from build123d import *

# Parameters (mm, degrees)
SKETCH1_R           = 14
BOSS_EXTRUDE1_DEPTH = 22
SKETCH2_R           = 12
CUT_EXTRUDE1_DEPTH  = 15
SKETCH3_R           = 17.036826926
SKETCH3_R_2         = 13
CUT_EXTRUDE2_DEPTH  = 15
SKETCH4_R           = 15.163293939
CUT_EXTRUDE3_DEPTH  = 10
SKETCH5_R           = 16.994892588
SKETCH5_R_2         = 4.5
CUT_EXTRUDE4_DEPTH  = 2
SKETCH8_R           = 3.6
CUT_EXTRUDE5_DEPTH  = 7
CIRPATTERN1_COUNT   = 4
SKETCH11_R          = 5.620004384
CUT_EXTRUDE6_DEPTH  = 0.75
SKETCH12_R          = 1.5
CUT_EXTRUDE7_DEPTH  = 18
SKETCH13_R          = 8.375
SKETCH13_R_2        = 4.775
CUT_EXTRUDE8_DEPTH  = 3
FILLET1_SIZE        = 2.75
FILLET2_SIZE        = 3
SKETCH14_W          = 4
SKETCH14_H          = 4.217169846
CUT_EXTRUDE10_DEPTH = 5
CIRPATTERN3_COUNT   = 14
CIRPATTERN3_ANGLE   = 334.282
SKETCH16_R          = 0.75
CUT_EXTRUDE11_DEPTH = 6


with BuildPart() as part:
    # Sketch1 → Boss-Extrude1 (new body)
    with BuildSketch(Plane.XY):
        Circle(SKETCH1_R)
    extrude(amount=BOSS_EXTRUDE1_DEPTH)

    # Sketch2 → Cut-Extrude1 (cut)
    with BuildSketch(Plane(origin=(0, 0, 0), x_dir=(-1, 0, 0), z_dir=(0, 0, -1))):
        Circle(SKETCH2_R)
    extrude(amount=-CUT_EXTRUDE1_DEPTH, mode=Mode.SUBTRACT)

    # Sketch3 → Cut-Extrude2 (cut)
    with BuildSketch(Plane(origin=(0, 0, 0), x_dir=(-1, 0, 0), z_dir=(0, 0, -1))):
        Circle(SKETCH3_R)
        Circle(SKETCH3_R_2, mode=Mode.SUBTRACT)
    extrude(amount=-CUT_EXTRUDE2_DEPTH, mode=Mode.SUBTRACT)

    # Sketch4 → Cut-Extrude3 (cut)
    with BuildSketch(Plane(origin=(0, 0, 0), x_dir=(-1, 0, 0), z_dir=(0, 0, -1))):
        Circle(SKETCH4_R)
    extrude(amount=-CUT_EXTRUDE3_DEPTH, mode=Mode.SUBTRACT)

    # Sketch5 → Cut-Extrude4 (cut)
    with BuildSketch(Plane.XY.offset(22)):
        Circle(SKETCH5_R)
        Circle(SKETCH5_R_2, mode=Mode.SUBTRACT)
    extrude(amount=-CUT_EXTRUDE4_DEPTH, mode=Mode.SUBTRACT)

    # Sketch8 → Cut-Extrude5 (cut)
    with BuildSketch(Plane.XY.offset(20)):
        with Locations((0, 8.375)):
            Circle(SKETCH8_R)
    cut_extrude5 = extrude(amount=-CUT_EXTRUDE5_DEPTH, mode=Mode.SUBTRACT)

    # CirPattern1: Cut-Extrude5 ×4 about axis
    cirpattern1_axis = Axis((0, 0, 0), (0, 0, 1))
    for i in range(1, CIRPATTERN1_COUNT):
        add(cut_extrude5.rotate(cirpattern1_axis, i * 360 / CIRPATTERN1_COUNT), mode=Mode.SUBTRACT)

    # Sketch7 → Cut-Revolve2 (revolve, cut)
    with BuildSketch(Plane(origin=(0, 0, 0), x_dir=(1, 0, 0), z_dir=(0, 1, 0))):
        with BuildLine():
            Line((-14, -16), (-16.211067118, -22.850526422))
            Line((-16.211067118, -22.850526422), (-8.5, -20))
            add(Edge.make_bspline(
                [(-8.5, -20), (-12.342847144, -17.893785877), (-14, -16)],
                knots=[0, 0, 0, 1, 1, 1], degree=2))
        make_face()
    revolve(axis=Axis((0, 0, 9.142490177), (0, 0, 1)), mode=Mode.SUBTRACT)

    # Sketch11 → Cut-Extrude6 (cut)
    with BuildSketch(Plane.XY.offset(22)):
        Circle(SKETCH11_R)
    extrude(amount=-CUT_EXTRUDE6_DEPTH, mode=Mode.SUBTRACT)

    # Sketch12 → Cut-Extrude7 (cut)
    with BuildSketch(Plane.XY.offset(21.25)):
        Circle(SKETCH12_R)
    extrude(amount=-CUT_EXTRUDE7_DEPTH, mode=Mode.SUBTRACT)

    # Sketch13 → Cut-Extrude8 (cut)
    with BuildSketch(Plane(origin=(0, 0, 15), x_dir=(-1, 0, 0), z_dir=(0, 0, -1))):
        Circle(SKETCH13_R)
        Circle(SKETCH13_R_2, mode=Mode.SUBTRACT)
    extrude(amount=-CUT_EXTRUDE8_DEPTH, mode=Mode.SUBTRACT)

    # Fillet1
    fillet1_edges = [part.edges().sort_by_distance(p)[0] for p in [
        (4.775, 0, 15),
    ]]
    chamfer(fillet1_edges, length=FILLET1_SIZE)

    # Fillet2
    # the kernel refuses this chamfer: 3 mm, written as the material it takes off along each edge
    with BuildSketch(Plane(origin=(0, 0, 15), x_dir=(-0.4688986407455129, 0.8832519825661364, 0), z_dir=(-0.8832519825661364, -0.4688986407455129, 0))) as fillet2_piece_1_section:
        Polygon((8.375, -FILLET2_SIZE), (8.375 + FILLET2_SIZE, 0), (8.375, 0), align=None)
    fillet2_piece_1 = revolve(axis=Axis((0, 0, 15), (0, 0, -1)), revolution_arc=145.925657294, mode=Mode.PRIVATE)
    fillet2_piece_1 = split(fillet2_piece_1, bisect_by=Plane(origin=(6.988160105, 6.988160105, 18), z_dir=(0, 0, -1)), keep=Keep.TOP, mode=Mode.PRIVATE)
    add(fillet2_piece_1, mode=Mode.SUBTRACT)
    with BuildSketch(Plane(origin=(0, 0, 15), x_dir=(0.4688986407455169, -0.8832519825661342, 0), z_dir=(0.8832519825661342, 0.4688986407455169, 0))) as fillet2_piece_2_section:
        Polygon((8.375, -FILLET2_SIZE), (8.375 + FILLET2_SIZE, 0), (8.375, 0), align=None)
    fillet2_piece_2 = revolve(axis=Axis((0, 0, 15), (0, 0, -1)), revolution_arc=145.925657294, mode=Mode.PRIVATE)
    fillet2_piece_2 = split(fillet2_piece_2, bisect_by=Plane(origin=(-6.988160104, -6.988160104, 18), z_dir=(0, 0, -1)), keep=Keep.TOP, mode=Mode.PRIVATE)
    add(fillet2_piece_2, mode=Mode.SUBTRACT)
    with BuildSketch(Plane(origin=(0, 0, 15), x_dir=(0.8832519825661352, 0.4688986407455149, 0), z_dir=(-0.4688986407455149, 0.8832519825661352, 0))) as fillet2_piece_3_section:
        Polygon((8.375, -FILLET2_SIZE), (8.375 + FILLET2_SIZE, 0), (8.375, 0), align=None)
    fillet2_piece_3 = revolve(axis=Axis((0, 0, 15), (0, 0, -1)), revolution_arc=145.925657294, mode=Mode.PRIVATE)
    fillet2_piece_3 = split(fillet2_piece_3, bisect_by=Plane(origin=(6.988160105, -6.988160105, 18), z_dir=(0, 0, -1)), keep=Keep.TOP, mode=Mode.PRIVATE)
    add(fillet2_piece_3, mode=Mode.SUBTRACT)
    with BuildSketch(Plane(origin=(0, 0, 15), x_dir=(-0.8832519825661325, -0.46889864074552023, 0), z_dir=(0.46889864074552023, -0.8832519825661325, 0))) as fillet2_piece_4_section:
        Polygon((8.375, -FILLET2_SIZE), (8.375 + FILLET2_SIZE, 0), (8.375, 0), align=None)
    fillet2_piece_4 = revolve(axis=Axis((0, 0, 15), (0, 0, -1)), revolution_arc=145.925657294, mode=Mode.PRIVATE)
    fillet2_piece_4 = split(fillet2_piece_4, bisect_by=Plane(origin=(-6.988160105, 6.988160105, 18), z_dir=(0, 0, -1)), keep=Keep.TOP, mode=Mode.PRIVATE)
    add(fillet2_piece_4, mode=Mode.SUBTRACT)

    # Sketch14 → Cut-Extrude10 (cut)
    with BuildSketch(Plane(origin=(0, 0, 10), x_dir=(-1, 0, 0), z_dir=(0, 0, -1))):
        with Locations((0, 13.940744489)):
            Rectangle(SKETCH14_W, SKETCH14_H)
    cut_extrude10 = extrude(amount=-CUT_EXTRUDE10_DEPTH, mode=Mode.SUBTRACT)

    # CirPattern3: Cut-Extrude10 ×14 about axis
    cirpattern3_axis = Axis((0, 0, 0), (0, 0, 1))
    for i in range(1, CIRPATTERN3_COUNT):
        add(cut_extrude10.rotate(cirpattern3_axis, i * CIRPATTERN3_ANGLE / (CIRPATTERN3_COUNT - 1)), mode=Mode.SUBTRACT)

    # Sketch16 → Cut-Extrude11 (cut)
    with BuildSketch(Plane(origin=(0, 0, 0), x_dir=(1, 0, 0), z_dir=(0, 1, 0))):
        with Locations(Location((0, -18.946648634, 0), (0, 0, 270))):
            Circle(SKETCH16_R)
    extrude(amount=-CUT_EXTRUDE11_DEPTH, mode=Mode.SUBTRACT)


solid = part.part
Geometry: final body of the model. Coordinates: model frame, mm. A direction names the side the tool comes from. Round coordinates to 2 decimals unless told otherwise and drop trailing zeros. Loops run counter-clockwise (first coordinate to the right, second up) from the corner with the lowest first, then second, coordinate; pieces in that order, holes last.
Q1. Access query for faces 1 (the cylindrical face through (-0.59, 4.46, 20.63)), 2 (the flat face through (-11.6, -4.7, 12.5)), 3 (the flat face through (-5, -4, 18)), 4 (the cylindrical face through (11.718, -5.63, 12.465)), 5 (the flat face through (7.15, -10.24, 12.46)). Directions: +Z, -Z, +X, -X, +Y, -Y. A direction counts if a zero-diameter tool reaches every point of the face in a straight line with its end or side. Return the directions, or none.
Q2. Section A-A on z = 12.25. State how many separate pieces and enclosed holes the cut face has, plus the area to 3 significant figures.
Q3. Pin query (flat end, axial travel): P1, Ø3, axis at x = 10, y = 1.5, coming from the -Z side; P2, Ø1, axis at x = -9, z = 12, coming from the -Y side; P3, Ø0.5, axis at y = -12.5, z = 13, coming from the -X side; P4, Ø6.5, axis at x = 0, y = 8.375, coming from the -Z side. Return the tip coordinate at first contact, or that it passes through.
Q4. Pull-direction query (X, two-part tool) for faces 6 (the cylindrical face through (-8.1, -10.17, 12.46)), 7 (the cylindrical face through (2.66, 11.7, 12.46)), 8 (the flat face through (0, -2, 21.25)); classes: released by +X, released by -X, zero draft, split by the parting line, or undercut.
Q5. Material intervals for L1, parallel to Y at x = 0, z = 17.35 (3 decimals); L2, parallel to Y at x = 0, z = 17.5 (3 decimals); L3, parallel to Y at x = -7.5, z = 10.5, sorted ascending.
Q6. Section B-B on z = 20.75. Return loops of the section in (x, y).
Evaluation:
1. face 1: +Z
1. face 2: -Z, -X
1. face 3: -Z
1. face 4: -Z, +X, -Y
1. face 5: -Z, -Y
2. separate pieces: 14
2. enclosed holes: 0
2. area: 22.3 mm2
3. P1: stops at z = 15
3. P2: stops at y = -9.84
3. P3: stops at x = -3.77
3. P4: passes through
4. face 6: released by -X
4. face 7: undercut
4. face 8: zero draft
5. L1: y = -12.574 to -11.975, -4.375 to -1.5, 1.5 to 4.375, 11.975 to 12.574
5. L2: y = -12.387 to -11.975, -4.525 to -1.5, 1.5 to 4.525, 11.975 to 12.387
5. L3: y = -10.62 to -9.37, 9.37 to 10.62
6. outline: circle Ø9 at (0, 0); hole circle Ø3 at (0, 0)
